CAD build for the part. Positions are in the model's coordinates, mm. A direction names the side the tool comes from. Round coordinates to 2 decimals unless told otherwise and drop trailing zeros. Loops run counter-clockwise (first coordinate to the right, second up) from the corner with the lowest first, then second, coordinate; pieces in that order, holes last. Notation, with made-up numbers: M 70,-20 L 108,-20 A13 ccw 108,-9 Z; hole C 67.5,-25.5 d4. An arc over 180 degrees is marked long. Use one line per item in the form item = value.
Autodesk Inventor part; units mm, degrees
ref_plane "YZ Plane" through (0, 0, 0) normal (1, 0, 0) x (0, 1, 0)
ref_plane "XZ Plane" through (0, 0, 0) normal (0, 1, 0) x (-1, 0, 0)
ref_plane "XY Plane" through (0, 0, 0) normal (0, 0, 1) x (1, 0, 0)
sketch "Эскиз1" plane through (0, 0, 0) normal (0, 0, 1) x (1, 0, 0)
  line L0 (-236.7799, 208.2081) -> (-236.7799, 188.2081)
  line L1 (-216.7799, 208.2081) -> (-236.7799, 208.2081)
  line L2 (-236.7799, 188.2081) -> (-235.1299, 188.2081)
  line L3 (-235.1299, 188.2081) -> (-235.1299, 206.5581)
  line L4 (-235.1299, 206.5581) -> (-216.7799, 206.5581)
  line L5 (-216.7799, 206.5581) -> (-216.7799, 208.2081)
  line L6 (-216.7799, 206.5581) -> (-216.7799, 201.4081)
  line L7 (-216.7799, 201.4081) -> (-229.9799, 188.2081)
  line L8 (-229.9799, 188.2081) -> (-235.1299, 188.2081)
  line L9 (-236.7799, 208.2081) -> (-223.3799, 194.8081) construction
  circle A0 centre (-226.7799, 198.2081) radius 2
  point P0 (0, 0)
  dimension "d0" = 20
  dimension "d1" = 20
  dimension "d2" = 1.65
  dimension "d3" = 1.65
  dimension "d6" = 6.8
  dimension "d7" = 6.8
  dimension "d10" = 4
  dimension "d11" = 10
extrude "Выдавливание1" add sketch "Эскиз1" along normal blind 353 contours L1 L5 L4 L3 L2 L0
extrude "Выдавливание2" add sketch "Эскиз1" along normal blind 1.65 contours L3 L4 L6 L7 L8 | A0
extrude "Выдавливание3" cut sketch "Эскиз1" along normal blind 1.65 contours A0
fillet "Сопряжение1" radius 2 1 edges at (-235.1299, 206.5581, 177.325)
fillet "Сопряжение2" radius 3.65 1 edges at (-236.7799, 208.2081, 176.5)
fillet "Сопряжение3" radius 3.65 3 edges at (-235.7109, 207.1391, 0) (-236.7799, 196.3831, 0) (-224.9549, 208.2081, 0)
fillet "Сопряжение4" radius 2 3 edges at (-234.5442, 205.9724, 1.65) (-235.1299, 196.3831, 1.65) (-224.9549, 206.5581, 1.65)
sketch "Эскиз2" plane through (-236.7799, 188.2081, 353) normal (-1, 0, 0) x (0, 0, 1)
  circle A0 centre (-344, 8.5) radius 1.5
  line L0 (-353, 16.35) -> (-353, 0)
  line L1 (-349.35, 0) -> (0, 0)
  circle A1 centre (-318.5, 8.5) radius 2
  circle A2 centre (-304.5, 8.5) radius 2
  line L2 (-318.5, 8.5) -> (-304.5, 8.5) construction
  circle A3 centre (-274, 5.5) radius 1.5
  circle A4 centre (-157, 8.5) radius 2
  circle A5 centre (-90, 8.5) radius 2
  circle A6 centre (-76, 8.5) radius 2
  line L3 (0, 16.35) -> (0, 0)
  circle A7 centre (-47, 8.5) radius 1.5
  circle A8 centre (-35, 8) radius 2
  circle A9 centre (-8, 10) radius 2
  point P0 (-353, -188.2081)
  dimension "d18" = 3
  dimension "d19" = 9
  dimension "d20" = 8.5
  dimension "d21" = 4
  dimension "d22" = 4
  dimension "d23" = 34.5
  dimension "d24" = 8.5
  dimension "d25" = 14
  dimension "d26" = 3
  dimension "d27" = 5.5
  dimension "d28" = 79
  dimension "d29" = 4
  dimension "d30" = 8.5
  dimension "d31" = 196
  dimension "d32" = 4
  dimension "d33" = 4
  dimension "d34" = 8.5
  dimension "d35" = 8.5
  dimension "d36" = 90
  dimension "d37" = 14
  dimension "d38" = 3
  dimension "d39" = 8.5
  dimension "d40" = 47
  dimension "d41" = 4
  dimension "d42" = 4
  dimension "d43" = 8
  dimension "d44" = 10
  dimension "d45" = 8
  dimension "d46" = 27
  dimension "d47" = 12
extrude "Выдавливание4" cut sketch "Эскиз2" against normal blind 1.65
sketch "Эскиз3" plane through (-233.1299, 208.2081, 353) normal (0, 1, 0) x (1, 0, 0)
  circle A0 centre (7.85, 344) radius 1.5
  line L0 (16.35, 353) -> (0, 353)
  line L1 (16.35, 349.35) -> (16.35, 0)
  circle A1 centre (8.35, 35) radius 2
  circle A2 centre (6.35, 8) radius 2
  line L2 (16.35, 0) -> (0, 0)
  circle A3 centre (7.85, 47) radius 1.5
  circle A4 centre (7.85, 129) radius 2
  circle A5 centre (7.85, 92) radius 2
  point P0 (233.1299, 353)
  dimension "d50" = 3
  dimension "d51" = 9
  dimension "d52" = 8.5
  dimension "d53" = 4
  dimension "d54" = 4
  dimension "d55" = 8
  dimension "d56" = 10
  dimension "d57" = 27
  dimension "d58" = 8
  dimension "d59" = 3
  dimension "d60" = 8.5
  dimension "d61" = 12
  dimension "d62" = 4
  dimension "d63" = 4
  dimension "d64" = 8.5
  dimension "d65" = 8.5
  dimension "d66" = 37
  dimension "d67" = 92
extrude "Выдавливание5" cut sketch "Эскиз3" against normal blind 1.65
sketch "Эскиз4" plane through (-233.1299, 208.2081, 353) normal (0, 1, 0) x (1, 0, 0)
  line L0 (13.85, 9) -> (16.35, 9)
  line L1 (16.35, 349.35) -> (16.35, 0)
  line L2 (16.35, 9) -> (16.35, 16)
  line L3 (16.35, 16) -> (13.85, 16)
  arc A0 (13.85, 16) -> (13.85, 9) centre (13.85, 12.5) ccw
  line L4 (16.35, 0) -> (0, 0)
  point P0 (233.1299, 353)
  dimension "d72" = 3.5
  dimension "d73" = 7
  dimension "d74" = 6
  dimension "d75" = 9
extrude "Выдавливание6" cut sketch "Эскиз4" against normal blind 10
sketch "Эскиз5" plane through (-236.7799, 188.2081, 353) normal (-1, 0, 0) x (0, 0, 1)
  arc A0 (-9, 2.5) -> (-16, 2.5) centre (-12.5, 2.5) ccw
  line L0 (-9, 2.5) -> (-9, 0)
  line L1 (-349.35, 0) -> (0, 0)
  line L2 (-9, 0) -> (-16, 0)
  line L3 (-16, 0) -> (-16, 2.5)
  line L4 (0, 16.35) -> (0, 0)
  point P0 (-353, -188.2081)
  dimension "d78" = 7
  dimension "d79" = 6
  dimension "d80" = 9
extrude "Выдавливание7" cut sketch "Эскиз5" against normal blind 10
properties part number "стойка"
1. Cut at A-A on z = 247.5. Write the cut outline in (x, y).
Completed:
outline = M -236.78,188.21 L -235.13,188.21 L -235.13,204.56 A2 cw -233.13,206.56 L -216.78,206.56 L -216.78,208.21 L -233.13,208.21 A3.65 ccw -236.78,204.56 Z
2. Tool access for faces 1 (the face through (-225, 208.208, 176)), 2 (the face through (-229, 200, 1.65)): list every direction of +Z, -Z, +X, -X, +Y, -Y with a clear straight run to the whole face (end or side of a thin tool).
Completed:
face_1 = +Z, -Z, +X, -X, +Y
face_2 = +Z, +X, -Y
3. Probe line 1 along Z through (x, y) = (-224.25, 201.75); line 2 along X through (y, z) = (190.5, 304); line 3 along Y through (x, z) = (-218.75, 237.5). List the from-to ranges inside material, lowest first. Write a range as from..to.
Completed:
line_1 = 0..1.65
line_2 = -236.78..-235.13
line_3 = 206.56..208.21
4. Drop flat-ended pins along their axis: P1, Ø8, axis at y = 193.5, z = 68.5, coming from the +X side; P2, Ø0.5, axis at x = -236, y = 189, coming from the -Z side; P3, Ø5, axis at y = 203.5, z = 75.5, coming from the +X side. Give the stop position or say it passes through.
Completed:
P1 = -235.13
P2 = 1.11
P3 = -234.52
